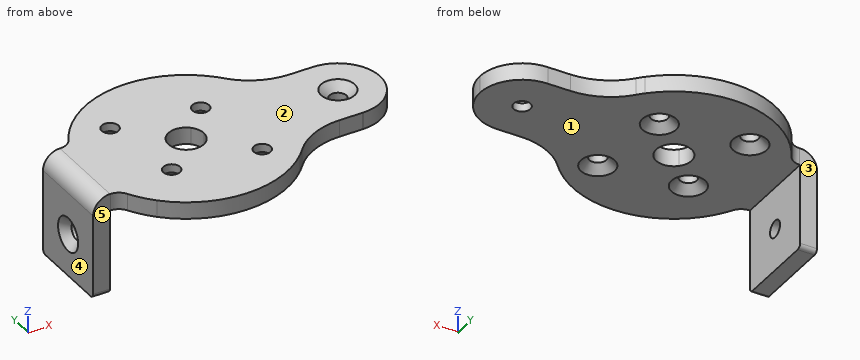
from build123d import *

# Parameters (mm, degrees)
F1_DEPTH        = 2
F3_DEPTH        = 5
F4_R            = 1.7
F5_R            = 1.7
F7_D            = 2
F7_CSINK_D      = 4
F7_CSINK_ANGLE  = 90
F8_DEPTH        = 2
F9_D            = 2
F9_CSINK_D      = 4
F9_CSINK_ANGLE  = 90
F10_R           = 0.5
F12_D           = 2
F12_CSINK_D     = 4
F12_CSINK_ANGLE = 90


with BuildPart() as f1:
    # F0 (on Top) → F1 (new body)
    with BuildSketch(Plane.XY):
        with BuildLine():
            ThreePointArc((10.9090595084, -4.9992420067), (11.7240930161, -2.5584454166), (12, 0))
            ThreePointArc((12, 0), (11.7240719072, 2.5585421465), (10.9089770141, 4.9994220172))
            ThreePointArc((10.9089770141, 4.9994220172), (10.1116451525, 6.4617824406), (9.1195071029, 7.7996532103))
            ThreePointArc((9.1195071029, 7.7996532103), (8.8090672506, 8.1486400199), (8.4852813742, 8.4852813742))
            Line((8.4852813742, 8.4852813742), (5.6568542495, 5.6568542495))
            ThreePointArc((5.6568542495, 5.6568542495), (7.3910362601, 3.0614674589), (8, 0))
            ThreePointArc((8, 0), (7.3910362601, -3.0614674589), (5.6568542495, -5.6568542495))
            Line((5.6568542495, -5.6568542495), (8.4852813742, -8.4852813742))
            ThreePointArc((8.4852813742, -8.4852813742), (8.8091155041, -8.1485878553), (9.1195994764, -7.799545204))
            ThreePointArc((9.1195994764, -7.799545204), (10.1117367293, -6.4616391356), (10.9090595084, -4.9992420067))
        make_face()
        with BuildLine():
            ThreePointArc((10.9089770141, 4.9994220172), (11.7240719072, 2.5585421465), (12, 0))
            ThreePointArc((12, 0), (11.7240930161, -2.5584454166), (10.9090595084, -4.9992420067))
            Line((10.9090595084, -4.9992420067), (15.1993324607, -4.9992420067))
            Line((15.1993324607, -4.9992420067), (17.9129404916, -4.9992420067))
            ThreePointArc((17.9129404916, -4.9992420067), (13.0000030459, 0.0055189952), (17.9239770141, 4.9994220172))
            Line((17.9239770141, 4.9994220172), (15.1991785048, 4.9994220172))
            Line((15.1991785048, 4.9994220172), (10.9089770141, 4.9994220172))
        make_face()
        with BuildLine():
            ThreePointArc((9.1195071029, 7.7996532103), (10.1116451525, 6.4617824406), (10.9089770141, 4.9994220172))
            Line((10.9089770141, 4.9994220172), (15.1991785048, 4.9994220172))
            ThreePointArc((15.1991785048, 4.9994220172), (11.8524002372, 5.7331248014), (9.1195071029, 7.7996532103))
        make_face()
        with BuildLine():
            Line((15.1993324607, -4.9992420067), (10.9090595084, -4.9992420067))
            ThreePointArc((10.9090595084, -4.9992420067), (10.1117367293, -6.4616391356), (9.1195994764, -7.799545204))
            ThreePointArc((9.1195994764, -7.799545204), (11.8525111644, -5.7329646097), (15.1993324607, -4.9992420067))
        make_face()
        with BuildLine():
            Line((5.6568542495, 5.6568542495), (8.4852813742, 8.4852813742))
            ThreePointArc((8.4852813742, 8.4852813742), (0, 12), (-8.4852813742, 8.4852813742))
            Line((-8.4852813742, 8.4852813742), (-5.6568542495, 5.6568542495))
            ThreePointArc((-5.6568542495, 5.6568542495), (0, 8), (5.6568542495, 5.6568542495))
        make_face()
        with BuildLine():
            ThreePointArc((23, 0), (21.5085527693, 3.5623106918), (17.9239770141, 4.9994220172))
            ThreePointArc((17.9239770141, 4.9994220172), (13.0000030459, 0.0055189952), (17.9129404916, -4.9992420067))
            Line((17.9129404916, -4.9992420067), (18.0870595084, -4.9992420067))
            ThreePointArc((18.0870595084, -4.9992420067), (21.5661812589, -3.5046185568), (23, 0))
        make_face()
        with BuildLine():
            ThreePointArc((-8.4852813742, -8.4852813742), (0, -12), (8.4852813742, -8.4852813742))
            Line((8.4852813742, -8.4852813742), (5.6568542495, -5.6568542495))
            ThreePointArc((5.6568542495, -5.6568542495), (0, -8), (-5.6568542495, -5.6568542495))
            Line((-5.6568542495, -5.6568542495), (-8.4852813742, -8.4852813742))
        make_face()
        with BuildLine():
            Line((18.0870595084, -4.9992420067), (17.9129404916, -4.9992420067))
            ThreePointArc((17.9129404916, -4.9992420067), (18, -5), (18.0870595084, -4.9992420067))
        make_face()
        with BuildLine():
            Line((-5.6568542495, 5.6568542495), (-8.4852813742, 8.4852813742))
            ThreePointArc((-8.4852813742, 8.4852813742), (-12, 0), (-8.4852813742, -8.4852813742))
            Line((-8.4852813742, -8.4852813742), (-5.6568542495, -5.6568542495))
            ThreePointArc((-5.6568542495, -5.6568542495), (-8, 0), (-5.6568542495, 5.6568542495))
        make_face()
    extrude(amount=F1_DEPTH)

    # F2 (on Front) → F3 (join, symmetric)
    with BuildSketch(Plane.XZ):
        with BuildLine():
            Line((-11.9999999998, -10), (-11.9999999998, 0))
            Line((-11.9999999998, 0), (-8.9999999998, 0))
            Line((-8.9999999998, 0), (-8.9999999998, 2))
            Line((-8.9999999998, 2), (-11.9999999998, 2))
            ThreePointArc((-11.9999999998, 2), (-13.4142135622, 1.4142135624), (-13.9999999998, 0))
            Line((-13.9999999998, 0), (-13.9999999998, -10))
            Line((-13.9999999998, -10), (-11.9999999998, -10))
        make_face()
    extrude(amount=F3_DEPTH, both=True)

    # F4
    f4_edges = [f1.edges().sort_by_distance(p)[0] for p in [
        (-10.908712, -5, 1),
    ]]
    fillet(f4_edges, radius=F4_R)

    # F5
    f5_edges = [f1.edges().sort_by_distance(p)[0] for p in [
        (-10.908712, 5, 1),
    ]]
    fillet(f5_edges, radius=F5_R)

    # F7 (through all)
    with Locations(Plane.XY.offset(2)):
        with Locations((18, 0)):
            CounterSinkHole(F7_D / 2, F7_CSINK_D / 2, counter_sink_angle=F7_CSINK_ANGLE)

    # F0 (on Top) → F8 (join)
    with BuildSketch(Plane.XY):
        with BuildLine():
            Line((-4.2426406871, 4.2426406871), (-5.6568542495, 5.6568542495))
            ThreePointArc((-5.6568542495, 5.6568542495), (-8, 0), (-5.6568542495, -5.6568542495))
            Line((-5.6568542495, -5.6568542495), (-4.2426406871, -4.2426406871))
            ThreePointArc((-4.2426406871, -4.2426406871), (-6, 0), (-4.2426406871, 4.2426406871))
        make_face()
        with BuildLine():
            Line((4.2426406871, 4.2426406871), (5.6568542495, 5.6568542495))
            ThreePointArc((5.6568542495, 5.6568542495), (0, 8), (-5.6568542495, 5.6568542495))
            Line((-5.6568542495, 5.6568542495), (-4.2426406871, 4.2426406871))
            ThreePointArc((-4.2426406871, 4.2426406871), (0, 6), (4.2426406871, 4.2426406871))
        make_face()
        with BuildLine():
            ThreePointArc((8, 0), (7.3910362601, 3.0614674589), (5.6568542495, 5.6568542495))
            Line((5.6568542495, 5.6568542495), (4.2426406871, 4.2426406871))
            ThreePointArc((4.2426406871, 4.2426406871), (5.5432771951, 2.2961005942), (6, 0))
            ThreePointArc((6, 0), (5.5432771951, -2.2961005942), (4.2426406871, -4.2426406871))
            Line((4.2426406871, -4.2426406871), (5.6568542495, -5.6568542495))
            ThreePointArc((5.6568542495, -5.6568542495), (7.3910362601, -3.0614674589), (8, 0))
        make_face()
        with BuildLine():
            ThreePointArc((6, 0), (5.5432771951, 2.2961005942), (4.2426406871, 4.2426406871))
            Line((4.2426406871, 4.2426406871), (1.4849242405, 1.4849242405))
            ThreePointArc((1.4849242405, 1.4849242405), (1.9401470183, 0.803635208), (2.1, 0))
            ThreePointArc((2.1, 0), (1.9401470183, -0.803635208), (1.4849242405, -1.4849242405))
            Line((1.4849242405, -1.4849242405), (4.2426406871, -4.2426406871))
            ThreePointArc((4.2426406871, -4.2426406871), (5.5432771951, -2.2961005942), (6, 0))
        make_face()
        with BuildLine():
            ThreePointArc((-4.2426406871, -4.2426406871), (0, -6), (4.2426406871, -4.2426406871))
            Line((4.2426406871, -4.2426406871), (1.4849242405, -1.4849242405))
            ThreePointArc((1.4849242405, -1.4849242405), (0, -2.1), (-1.4849242405, -1.4849242405))
            Line((-1.4849242405, -1.4849242405), (-4.2426406871, -4.2426406871))
        make_face()
        with BuildLine():
            Line((-1.4849242405, 1.4849242405), (-4.2426406871, 4.2426406871))
            ThreePointArc((-4.2426406871, 4.2426406871), (-6, 0), (-4.2426406871, -4.2426406871))
            Line((-4.2426406871, -4.2426406871), (-1.4849242405, -1.4849242405))
            ThreePointArc((-1.4849242405, -1.4849242405), (-2.1, 0), (-1.4849242405, 1.4849242405))
        make_face()
        with BuildLine():
            Line((1.4849242405, 1.4849242405), (4.2426406871, 4.2426406871))
            ThreePointArc((4.2426406871, 4.2426406871), (0, 6), (-4.2426406871, 4.2426406871))
            Line((-4.2426406871, 4.2426406871), (-1.4849242405, 1.4849242405))
            ThreePointArc((-1.4849242405, 1.4849242405), (0, 2.1), (1.4849242405, 1.4849242405))
        make_face()
        with BuildLine():
            ThreePointArc((-5.6568542495, -5.6568542495), (0, -8), (5.6568542495, -5.6568542495))
            Line((5.6568542495, -5.6568542495), (4.2426406871, -4.2426406871))
            ThreePointArc((4.2426406871, -4.2426406871), (0, -6), (-4.2426406871, -4.2426406871))
            Line((-4.2426406871, -4.2426406871), (-5.6568542495, -5.6568542495))
        make_face()
    extrude(amount=F8_DEPTH)

    # F9 (through all)
    with Locations(Plane(origin=(0, 0, 0), x_dir=(1, 0, 0), z_dir=(0, 0, -1))):
        with Locations((-4.2426406871, 4.2426406871), (5.6568542495, 5.6568542495), (4.2426406871, -4.2426406871), (-5.6568542495, -5.6568542495)):
            CounterSinkHole(F9_D / 2, F9_CSINK_D / 2, counter_sink_angle=F9_CSINK_ANGLE)

    # F10
    f10_edges = [f1.edges().sort_by_distance(p)[0] for p in [
        (-13, -5, -10),
        (-13, 5, -10),
    ]]
    fillet(f10_edges, radius=F10_R)

    # F12 (through all)
    with Locations(Plane(origin=(-13.9999999998, 0, 0), x_dir=(0, -1, 0), z_dir=(-1, 0, 0))):
        with Locations((0, -5)):
            CounterSinkHole(F12_D / 2, F12_CSINK_D / 2, counter_sink_angle=F12_CSINK_ANGLE)


solid = f1.part
Work out the finished part from the listing and answer in its coordinate system (mm). Face numbers are marked on the shaded views. A direction names the side the tool comes from. Give positions to 0.01 mm unless a question says otherwise; leave off trailing zeros. Order: outer loops, then holes, each group sorted by start corner. A loop starts at its lowest first (then second) coordinate and runs counter-clockwise, first axis right, second up. Notation, with made-up numbers: (54.5, -4.75) - (58.5, -4.75) arc R28 ccw to (58.5, 30.25) - close; hole circle Ø3 at (-22, 68). An arc over 180 degrees is marked (long way). Answer as CSV lines item,"result". Start each with the question number.
Q1. For the marked faces 1, 2, 3, 4 and 5, determine the directions among +Z, -Z, +X, -X, +Y, -Y from which every point of the face is accessible in a straight line to the end or side of a thin tool.
Q2. Given pin 1 Ø1.6 at (x, z) = (16.5, 0.5) entering from +Y; pin 2 Ø2.5 at (x, y) = (-5.66, 5.66) entering from +Z; pin 3 Ø1.6 at (x, y) = (18, 0) entering from -Z; pin 4 Ø0.6 at (x, z) = (-13, -4) entering from -Y, each flat-ended and moving along its own axis, determine where each tip first touches the part or whether it passes through.
Q3. The part is cut by section A-A (z = -5). Write down the section's boundary in (x, y), then the cut area to 3 significant figures.
Q4. The part is cut by section D-D (y = 0.5). Give the number of separate pieces and of enclosed holes in the cut face, then the cut area to 3 significant figures.
Q5. Find the intervals of material crossed by L1, parallel to Y at x = 18, z = 0.8; L2, parallel to Z at x = -10, y = -3.5; L3, parallel to X at y = -2.5, z = -1.5, in increasing order. Write a range as [from, to].
Q6. The part is cut by section C-C (z = -8). Write down the section's boundary in (x, y), then the cut area to 3 significant figures.
Q7. The part is cut by section B-B (y = 10.25). Write down the section's boundary in (x, z), then the cut area to 3 significant figures.
Check result:
1,face 1,"-Z, +X, +Y, -Y"
1,face 2,"+Z, +X, -X, +Y, -Y"
1,face 3,"+Z, -Z, -X, +Y"
1,face 4,"+Z, -Z, -X, +Y, -Y"
1,face 5,"+Z, -Z, -X, -Y"
2,pin 1,"stops at y = 5"
2,pin 2,"stops at z = 2"
2,pin 3,"passes through"
2,pin 4,"stops at y = -5"
3,outline,"(-14, -5) - (-12, -5) - (-12, -1) - (-13, -1) - (-14, -2) - close; (-14, 2) - (-13, 1) - (-12, 1) - (-12, 5) - (-14, 5) - close"
3,area,"15.0 mm²"
4,separate pieces,"4"
4,enclosed holes,"0"
4,area,"75.8 mm²"
5,L1,"y = [-5, -1], [1, 5]"
5,L2,"z = [0, 2]"
5,L3,"x = [-14, -12]"
6,outline,"(-14, -5) - (-12, -5) - (-12, 5) - (-14, 5) - close"
6,area,"20.0 mm²"
7,outline,"(-6.24, 0) - (6.24, 0) - (6.24, 2) - (-6.24, 2) - close"
7,area,"25.0 mm²"
